Read the model definition and answer for the solid it produces. Units are mm, in the model's axes. Round coordinates to 2 decimals unless told otherwise and drop trailing zeros. Loops run counter-clockwise (first coordinate to the right, second up) from the corner with the lowest first, then second, coordinate; pieces in that order, holes last. Notation, with made-up numbers: (24, 25.25) - (33, 25.25) arc R25 cw to (33, 40.25) - close; hole circle Ø7 at (3.5, 59.5). An arc over 180 degrees is marked (long way). Use CSV: the item, a comma, the result in double quotes. Start each with the question number.
1. Find section A-A (x = -1.5). Give the vertices of the cut face in (y, z).
2. Find section C-C (z = 5.5). Give the vertices of the cut face in (x, y).
3. Consider line 1 along Y through (x, z) = (0, 3); line 2 along X through (y, z) = (2.75, 4.75); line 3 along Y through (x, z) = (-22, 4.25). Determine where each line is inside the solid, lowest interval first.
4. Find section D-D (y = 9.25). Give the vertices of the cut face in (x, z), and give its area (3 significant figures).
5. Find section B-B (y = 0). Give the vertices of the cut face in (x, z).
6. Determine the mould class of faces 1 (the flat face through (-35, -12.5, 3.1)), 2 (the cylindrical face through (26.8, -2.4, 3.1)), 3 (the flat face through (8, 0, 0)) for opening direction X: +X half, -X half, draft (parallel to the pull), parting line (faces both ways), or undercut.
from build123d import *

# Parameters (mm, degrees)
SKETCH1_W           = 75
SKETCH1_H           = 30
SKETCH1_R           = 11
SKETCH1_R_2         = 2.5
SKETCH1_R_3         = 4
BOSS_EXTRUDE1_DEPTH = 6.35
CHAMFER1_SIZE       = 5


with BuildPart() as part:
    # Sketch1 → Boss-Extrude1 (new body)
    with BuildSketch(Plane.XY):
        Rectangle(SKETCH1_W, SKETCH1_H)
        with Locations((-22, 0)):
            Circle(SKETCH1_R, mode=Mode.SUBTRACT)
        Circle(SKETCH1_R_2, mode=Mode.SUBTRACT)
        with Locations((30, 0)):
            Circle(SKETCH1_R_3, mode=Mode.SUBTRACT)
    extrude(amount=BOSS_EXTRUDE1_DEPTH)

    # Chamfer1
    chamfer1_edges = [part.edges().sort_by_distance(p)[0] for p in [
        (37.5, -15, 3.175),
        (-37.5, -15, 3.175),
        (-37.5, 15, 3.175),
        (37.5, 15, 3.175),
    ]]
    chamfer(chamfer1_edges, length=CHAMFER1_SIZE)


solid = part.part
Filled sheet:
1,outline,"(-15, 0) - (-2, 0) - (-2, 6.35) - (-15, 6.35) - close; (2, 0) - (15, 0) - (15, 6.35) - (2, 6.35) - close"
2,outline,"(-37.5, -10) - (-32.5, -15) - (32.5, -15) - (37.5, -10) - (37.5, 10) - (32.5, 15) - (-32.5, 15) - (-37.5, 10) - close; hole circle Ø22 at (-22, 0); hole circle Ø5 at (0, 0); hole circle Ø8 at (30, 0)"
3,line 1,"y = -15 to -2.5, 2.5 to 15"
3,line 2,"x = -37.5 to -32.65, -11.35 to 27.1, 32.9 to 37.5"
3,line 3,"y = -15 to -11, 11 to 15"
4,outline,"(-37.5, 0) - (-27.95, 0) - (-27.95, 6.35) - (-37.5, 6.35) - close; (-16.05, 0) - (37.5, 0) - (37.5, 6.35) - (-16.05, 6.35) - close"
4,area,"401 mm²"
5,outline,"(-37.5, 0) - (-33, 0) - (-33, 6.35) - (-37.5, 6.35) - close; (-11, 0) - (-2.5, 0) - (-2.5, 6.35) - (-11, 6.35) - close; (2.5, 0) - (26, 0) - (26, 6.35) - (2.5, 6.35) - close; (34, 0) - (37.5, 0) - (37.5, 6.35) - (34, 6.35) - close"
6,face 1,"-X half"
6,face 2,"undercut"
6,face 3,"draft"
